from build123d import *

# Parameters (mm, degrees)
SKETCH1_W                                 = 60
SKETCH1_H                                 = 120
BOSS_EXTRUDE1_DEPTH                       = 12.7
SKETCH2_W                                 = 34.6
SKETCH2_H                                 = 7.7
CUT_EXTRUDE1_DEPTH                        = 121
F_3_32_0_09375_DIAMETER_HOLE1_D           = 2.38125
F_3_32_0_09375_DIAMETER_HOLE1_DEPTH       = 19.05
F_3_32_0_09375_DIAMETER_HOLE1_CSINK_D     = 3.175
F_3_32_0_09375_DIAMETER_HOLE1_CSINK_ANGLE = 90
F_3_32_0_09375_DIAMETER_HOLE1_TIP         = 0.715399675
CUT_EXTRUDE2_DEPTH                        = 1
CUT_EXTRUDE2_DEPTH_BACK                   = 121
F_5_16_18_TAPPED_HOLE1_D                  = 6.5278
F_5_16_18_TAPPED_HOLE1_DEPTH              = 32.45
F_5_16_18_TAPPED_HOLE1_CSINK_D            = 9.2075
F_5_16_18_TAPPED_HOLE1_CSINK_ANGLE        = 90
F_5_16_18_TAPPED_HOLE1_TIP                = 1.961148974
CHAMFER1_SIZE                             = 3.175
SKETCH6_W                                 = 15.1
SKETCH6_H                                 = 7.75
CUT_EXTRUDE3_DEPTH                        = 6
FILLET1_R                                 = 1
SKETCH7_R                                 = 2.8
CUT_EXTRUDE4_DEPTH                        = 6.0000001
CHAMFER2_SIZE                             = 2
SKETCH10_W                                = 60
SKETCH10_H                                = 100.95
CUT_EXTRUDE5_DEPTH                        = 7.7
SKETCH12_W                                = 24.87086649
SKETCH12_H                                = 0.4
CUT_EXTRUDE11_DEPTH                       = 121.0000001
SKETCH13_W                                = 34.6
SKETCH13_H                                = 0.374910819
CUT_EXTRUDE12_DEPTH                       = 121


with BuildPart() as part:
    # Sketch1 → Boss-Extrude1 (new body)
    with BuildSketch(Plane(origin=(0, 0, 0), x_dir=(1, 0, 0), z_dir=(0, 1, 0))):
        with Locations((0, 60)):
            Rectangle(SKETCH1_W, SKETCH1_H)
    extrude(amount=BOSS_EXTRUDE1_DEPTH)

    # Sketch2 → Cut-Extrude1 (cut, through all)
    with BuildSketch(Plane.XY):
        with Locations((0, 8.85)):
            Rectangle(SKETCH2_W, SKETCH2_H)
    extrude(amount=-CUT_EXTRUDE1_DEPTH, mode=Mode.SUBTRACT)

    # 3_32 _0.09375_ Diameter Hole1
    with Locations(Plane.XY):
        with Locations((0, 2.61875)):
            CounterSinkHole(F_3_32_0_09375_DIAMETER_HOLE1_D / 2, F_3_32_0_09375_DIAMETER_HOLE1_CSINK_D / 2, depth=F_3_32_0_09375_DIAMETER_HOLE1_DEPTH, counter_sink_angle=F_3_32_0_09375_DIAMETER_HOLE1_CSINK_ANGLE)
            with Locations((0, 0, -(F_3_32_0_09375_DIAMETER_HOLE1_DEPTH + F_3_32_0_09375_DIAMETER_HOLE1_TIP / 2))):  # 118° drill point
                Cone(0, F_3_32_0_09375_DIAMETER_HOLE1_D / 2, F_3_32_0_09375_DIAMETER_HOLE1_TIP, mode=Mode.SUBTRACT)

    # Sketch3 → Cut-Extrude2 (cut, two sides)
    with BuildSketch(Plane.XY) as cut_extrude2_sk:
        with BuildLine():
            Line((-124.818289263, -9.651397294), (-17.3, 0))
            ThreePointArc((-17.3, 0), (0, 0.774910819), (17.3, 0))
            Line((17.3, 0), (124.818289263, -9.651397294))
            Line((124.818289263, -9.651397294), (124.818289263, -225.552596882))
            Line((124.818289263, -225.552596882), (-124.818289263, -225.552596882))
            Line((-124.818289263, -225.552596882), (-124.818289263, -9.651397294))
        make_face()
    extrude(amount=CUT_EXTRUDE2_DEPTH, mode=Mode.SUBTRACT)
    extrude(cut_extrude2_sk.sketch, amount=-CUT_EXTRUDE2_DEPTH_BACK, mode=Mode.SUBTRACT)

    # 5_16-18 Tapped Hole1
    with Locations(Plane.XY):
        with Locations((-23.65, 6.35), (23.65, 6.35)):
            CounterSinkHole(F_5_16_18_TAPPED_HOLE1_D / 2, F_5_16_18_TAPPED_HOLE1_CSINK_D / 2, depth=F_5_16_18_TAPPED_HOLE1_DEPTH, counter_sink_angle=F_5_16_18_TAPPED_HOLE1_CSINK_ANGLE)
            with Locations((0, 0, -(F_5_16_18_TAPPED_HOLE1_DEPTH + F_5_16_18_TAPPED_HOLE1_TIP / 2))):  # 118° drill point
                Cone(0, F_5_16_18_TAPPED_HOLE1_D / 2, F_5_16_18_TAPPED_HOLE1_TIP, mode=Mode.SUBTRACT)

    # Chamfer1
    chamfer1_edges = [part.edges().sort_by_distance(p)[0] for p in [
        (-17.3, 12.7, -60),
        (17.3, 12.7, -60),
    ]]
    chamfer(chamfer1_edges, length=CHAMFER1_SIZE)

    # Sketch6 → Cut-Extrude3 (cut, through all)
    with BuildSketch(Plane(origin=(0, 5, 0), x_dir=(1, 0, 0), z_dir=(0, 1, 0))):
        with Locations((3.55, 107.9216)):
            Rectangle(SKETCH6_W, SKETCH6_H)
        with Locations((-2.75, 47.6216)):
            Rectangle(SKETCH6_W, SKETCH6_H)
    extrude(amount=-CUT_EXTRUDE3_DEPTH, mode=Mode.SUBTRACT)

    # Fillet1
    fillet1_edges = [part.edges().sort_by_distance(p)[0] for p in [
        (11.1, 2.72813819, -111.7966),
        (11.1, 2.72813819, -104.0466),
        (-4, 2.866781366, -104.0466),
        (-4, 2.866781366, -111.7966),
        (4.8, 2.857683387, -51.4966),
        (4.8, 2.857683387, -43.7466),
        (-10.3, 2.750290995, -43.7466),
        (-10.3, 2.750290995, -51.4966),
    ]]
    fillet(fillet1_edges, radius=FILLET1_R)

    # Sketch7 → Cut-Extrude4 (cut, through all)
    with BuildSketch(Plane(origin=(0, 5, 0), x_dir=(1, 0, 0), z_dir=(0, 1, 0))):
        with Locations(Location((-2.8, 64.7568, 0), (0, 0, 270))):  # turned: the seam where the file's is
            Circle(SKETCH7_R)
        with Locations(Location((0.3851, 25.9568, 0), (0, 0, 270))):  # turned: the seam where the file's is
            Circle(SKETCH7_R)
    extrude(amount=-CUT_EXTRUDE4_DEPTH, mode=Mode.SUBTRACT)

    # Chamfer2
    chamfer2_edges = [part.edges().sort_by_distance(p)[0] for p in [
        (3.55, 5, -104.0466),
        (-4, 5, -107.9216),
        (11.1, 5, -107.9216),
        (3.55, 5, -111.7966),
        (-2.75, 5, -51.4966),
        (4.8, 5, -47.6216),
        (-2.75, 5, -43.7466),
        (-10.3, 5, -47.6216),
        (-3.707106781, 5, -104.339493219),
        (10.807106781, 5, -104.339493219),
        (10.807106781, 5, -111.503706781),
        (4.507106781, 5, -51.203706781),
        (4.507106781, 5, -44.039493219),
        (-10.007106781, 5, -44.039493219),
        (-10.007106781, 5, -51.203706781),
        (-3.707106781, 5, -111.503706781),
        (-2.8, 5, -67.5568),
        (0.3851, 5, -28.7568),
    ]]
    chamfer(chamfer2_edges, length=CHAMFER2_SIZE)

    # Sketch10 → Cut-Extrude5 (cut)
    with BuildSketch(Plane(origin=(0, 12.7, 0), x_dir=(1, 0, 0), z_dir=(0, 1, 0))):
        with Locations((0, 69.525)):
            Rectangle(SKETCH10_W, SKETCH10_H)
    extrude(amount=-CUT_EXTRUDE5_DEPTH, mode=Mode.SUBTRACT)

    # Sketch12 → Cut-Extrude11 (cut, through all)
    with BuildSketch(Plane.XY):
        with Locations((0, 0.574910819)):
            Rectangle(SKETCH12_W, SKETCH12_H)
    extrude(amount=-CUT_EXTRUDE11_DEPTH, mode=Mode.SUBTRACT)

    # Sketch13 → Cut-Extrude12 (cut, through all)
    with BuildSketch(Plane.XY):
        with Locations((0, 0.18745541)):
            Rectangle(SKETCH13_W, SKETCH13_H)
    extrude(amount=-CUT_EXTRUDE12_DEPTH, mode=Mode.SUBTRACT)


solid = part.part
Could you check a few things on this model? Use its own coordinates, in mm. A direction names the side the tool comes from. Give positions to 0.01 mm unless a question says otherwise; leave off trailing zeros. Write each loop counter-clockwise with the first axis right and the second up, starting at its lowest first coordinate (ties: lowest second). Pieces come first, ordered by that corner, then holes. Notation, with made-up numbers: (-14, 49) -> (37, 49) arc R21 ccw to (37, 83) -> close; hole circle Ø5 at (-29, 49). An arc over 180 degrees is marked (long way). Answer as CSV lines item,"result". Start each with the question number.
(1) If we section it at A-A, the plane x = 23.65: Write out the boundary of the cut face in (y, z).
(2) If we mould it in two halves opening along Y, with no side actions, what happens to faces 1 (the face through (0.15, 3.8, -9.85)), 2 (the face through (15, 0.375, -59)), 3 (the face through (30, 3, -59))? For each: +Y half, -Y half, draft (parallel to the pull), parting line (faces both ways), or undercut.
(3) Which directions (+Z, -Z, +X, -X, +Y, -Y) give clear straight access to the entire face, cutting with the end or side of a thin tool? Please do faces 4 (the face through (-15, 0.375, -59)), 5 (the face through (-4, 2, -108)), 6 (the face through (5.22, 3.986, -43.358)), 7 (the face through (18.91, 11.135, -9.392)).
(4) I'm going to push flat-ended pins straight in: pin 1 Ø10 at (x, z) = (-14.5, -27.5) entering from +Y; pin 2 Ø2.5 at (x, z) = (14, -57) entering from -Y; pin 3 Ø0.7 at (x, y) = (-1.5, 1.5) entering from +Z; pin 4 Ø12 at (x, z) = (-3, -79) entering from -Y. Where does each tip first touch, or does it pass through?
(5) If we section it at C-C, the plane z = -48: Write out the boundary of the cut face in (x, y), and give its area (3 significant figures).
(6) If we section it at B-B, the plane y = 6.35: Write out the boundary of the cut face in (x, z).
(7) Please list where these lines run through material, in increasing order: line 1 (X direction, y = 6.35, z = -9); line 2 (X direction, y = 1.5, z = -26.5); line 3 (Y direction, x = -22, z = -62).
(8) If we section it at D-D, the plane z = -96.5: Write out the boundary of the cut face in (x, y).
Answer list:
1,outline,"(0, -120) -> (5, -120) -> (5, -33.6) -> (3.09, -32.45) -> (3.09, -1.34) -> (1.75, 0) -> (0, 0) -> close; (9.61, -19.05) -> (12.7, -19.05) -> (12.7, 0) -> (10.95, 0) -> (9.61, -1.34) -> close"
2,face 1,"undercut"
2,face 2,"-Y half"
2,face 3,"draft"
3,face 4,"+Z, -Z, -Y"
3,face 5,"+Y, -Y"
3,face 6,"+Y"
3,face 7,"+Z, -Z, +Y"
4,pin 1,"y = 5"
4,pin 2,"y = 0.37"
4,pin 3,"z = 0"
4,pin 4,"y = 0.77"
5,outline,"(-30, 0) -> (-17.3, 0) -> (-17.3, 0.37) -> (-12.44, 0.37) -> (-12.44, 0.77) -> (-10.3, 0.77) -> (-10.3, 3) -> (-12.3, 5) -> (-30, 5) -> close; (4.8, 0.77) -> (12.44, 0.77) -> (12.44, 0.37) -> (17.3, 0.37) -> (17.3, 0) -> (30, 0) -> (30, 5) -> (6.8, 5) -> (4.8, 3) -> close"
5,area,"209 mm^2"
6,outline,"(-30, -19.05) -> (-26.91, -19.05) -> (-26.91, -1.34) -> (-28.25, 0) -> (-30, 0) -> close; (-20.39, -19.05) -> (-17.3, -19.05) -> (-17.3, 0) -> (-19.05, 0) -> (-20.39, -1.34) -> close; (17.3, -19.05) -> (20.39, -19.05) -> (20.39, -1.34) -> (19.05, 0) -> (17.3, 0) -> close; (26.91, -19.05) -> (30, -19.05) -> (30, 0) -> (28.25, 0) -> (26.91, -1.34) -> close"
7,line 1,"-30 to -26.91, -20.39 to -17.3, 17.3 to 20.39, 26.91 to 30"
7,line 2,"-30 to -2.36, 3.13 to 30"
7,line 3,"0 to 5"
8,outline,"(-30, 0) -> (-17.3, 0) -> (-17.3, 0.37) -> (-12.44, 0.37) -> (-12.44, 0.77) -> (12.44, 0.77) -> (12.44, 0.37) -> (17.3, 0.37) -> (17.3, 0) -> (30, 0) -> (30, 5) -> (-30, 5) -> close"
